Source: CAD feature listing. Evaluate the final solid. Frame: model axes, mm. A direction names the side the tool comes from. Give positions to 0.01 mm unless a question says otherwise; leave off trailing zeros. Loops run counter-clockwise (first coordinate to the right, second up) from the corner with the lowest first, then second, coordinate; pieces in that order, holes last. Notation, with made-up numbers: M 82,-6.75 L 110,-6.75 A18 cw 110,7.25 Z; hole C -1,55.5 d11. An arc over 180 degrees is marked long. Write item = value, one per line.
from build123d import *

# Parameters (mm, degrees)
ESQUISSE3_W             = 28
ESQUISSE3_H             = 20
BOSS_EXTRU_1_DEPTH      = 8
ESQUISSE4_W             = 22
ESQUISSE4_H             = 14
ENL_V_MAT_EXTRU_1_DEPTH = 6
ESQUISSE5_W             = 22
ESQUISSE5_H             = 3
ENL_V_MAT_EXTRU_2_DEPTH = 4
ESQUISSE7_R             = 1
BOSS_EXTRU_2_DEPTH      = 5
ESQUISSE9_R             = 1
ENL_V_MAT_EXTRU_3_DEPTH = 2
ESQUISSE11_R            = 1
ENL_V_MAT_EXTRU_4_DEPTH = 2


with BuildPart() as part:
    # Esquisse3 → Boss.-Extru.1 (new body)
    with BuildSketch(Plane(origin=(0, 0, 0), x_dir=(1, 0, 0), z_dir=(0, 1, 0))):
        with Locations((-14, -10)):
            Rectangle(ESQUISSE3_W, ESQUISSE3_H)
    extrude(amount=BOSS_EXTRU_1_DEPTH)

    # Esquisse4 → Enlèv. mat.-Extru.1 (cut)
    with BuildSketch(Plane(origin=(0, 8, 0), x_dir=(1, 0, 0), z_dir=(0, 1, 0))):
        with Locations((-14, -10)):
            Rectangle(ESQUISSE4_W, ESQUISSE4_H)
    extrude(amount=-ENL_V_MAT_EXTRU_1_DEPTH, mode=Mode.SUBTRACT)

    # Esquisse5 → Enlèv. mat.-Extru.2 (cut)
    with BuildSketch(Plane(origin=(0, 8, 0), x_dir=(1, 0, 0), z_dir=(0, 1, 0))):
        with Locations((-14, -18.5)):
            Rectangle(ESQUISSE5_W, ESQUISSE5_H)
    extrude(amount=-ENL_V_MAT_EXTRU_2_DEPTH, mode=Mode.SUBTRACT)

    # Esquisse7 → Boss.-Extru.2 (add)
    with BuildSketch(Plane(origin=(0, 2, 0), x_dir=(1, 0, 0), z_dir=(0, 1, 0))):
        with Locations(Location((-14, -6, 0), (0, 0, 270))):
            Circle(ESQUISSE7_R)
    extrude(amount=BOSS_EXTRU_2_DEPTH)

    # Esquisse9 → Enlèv. mat.-Extru.3 (cut)
    with BuildSketch(Plane(origin=(0, 8, 0), x_dir=(1, 0, 0), z_dir=(0, 1, 0))):
        with Locations(Location((-26.25, -1.75, 0), (0, 0, 270))):
            Circle(ESQUISSE9_R)
    enl_v_mat_extru_3 = extrude(amount=-ENL_V_MAT_EXTRU_3_DEPTH, mode=Mode.SUBTRACT)

    # Symétrie1: Enlèv. mat.-Extru.3 across plane
    add(enl_v_mat_extru_3.mirror(Plane.ZY.offset(14)), mode=Mode.SUBTRACT)

    # Esquisse11 → Enlèv. mat.-Extru.4 (cut)
    with BuildSketch(Plane(origin=(0, 8, 0), x_dir=(1, 0, 0), z_dir=(0, 1, 0))):
        with Locations(Location((-26.5, -17.5, 0), (0, 0, 270))):
            Circle(ESQUISSE11_R)
    enl_v_mat_extru_4 = extrude(amount=-ENL_V_MAT_EXTRU_4_DEPTH, mode=Mode.SUBTRACT)

    # Symétrie2: Enlèv. mat.-Extru.4 across plane
    add(enl_v_mat_extru_4.mirror(Plane.ZY.offset(14)), mode=Mode.SUBTRACT)


solid = part.part
1. First-contact query: pin 1 Ø1.6 at (x, z) = (-26, 17.5) entering from +Y; pin 2 Ø3.5 at (x, z) = (-10.5, 18) entering from +Y; pin 3 Ø1.6 at (x, z) = (-26.25, 1.75) entering from +Y; pin 4 Ø7 at (x, z) = (-11.5, 13) entering from +Y. Flat tips, straight axial feed; report the tip coordinate or a pass-through.
Derived:
pin_1 = 8
pin_2 = 4
pin_3 = 6
pin_4 = 2
2. Cut plane C-C, the plane z = 1.75. Return the cut outline in (x, y), then the cut area to 3 significant figures.
Derived:
outline = M -28,0 L 0,0 L 0,8 L -0.75,8 L -0.75,6 L -2.75,6 L -2.75,8 L -25.25,8 L -25.25,6 L -27.25,6 L -27.25,8 L -28,8 Z
area = 216 mm²
3. Material intervals for probe 1 along X at (y, z) = (7, 17.5); probe 2 along X at (y, z) = (5.25, 18.5); probe 3 along X at (y, z) = (6.9, 1.75), sorted ascending. Write a range as from..to.
Derived:
probe_1 = -28..-27.5, -25.5..-25, -3..-2.5, -0.5..0
probe_2 = -28..-25, -3..0
probe_3 = -28..-27.25, -25.25..-2.75, -0.75..0
4. Pull-direction query (X, two-part tool) for faces 4 (the flat face through (-13, 8, 2.5)), 5 (the flat face through (-14, 3, 17)), 6 (the flat face through (0, 4, 10)); classes: +X half, -X half, draft (parallel to the pull), parting line (faces both ways), or undercut.
Derived:
face_4 = draft
face_5 = undercut
face_6 = +X half
5. Cut plane B-B, the plane x = -20.5. Return the cut outline in (y, z), then the cut area to 3 significant figures.
Derived:
outline = M 0,0 L 8,0 L 8,3 L 2,3 L 2,17 L 4,17 L 4,20 L 0,20 Z
area = 64.0 mm²
6. Cut plane D-D, the plane x = -14. Return the cut outline in (y, z), then the cut area to 3 significant figures.
Derived:
outline = M 0,0 L 8,0 L 8,3 L 2,3 L 2,5 L 7,5 L 7,7 L 2,7 L 2,17 L 4,17 L 4,20 L 0,20 Z
area = 74.0 mm²
7. Reachability of faces 1 (the flat face through (-25, 5, 12)), 2 (the flat face through (-14, 3, 20)), 3 (the flat face through (-14, 7, 6)) from +Z, -Z, +X, -X, +Y, -Y: full face, straight path, thin tool, end or side. Return the list, or none.
Derived:
face_1 = +Y
face_2 = +Z, +X, -X, +Y, -Y
face_3 = +Z, +Y
8. Cut plane A-A, the plane y = 2.5. Return the cut outline in (x, z).
Derived:
outline = M -28,0 L 0,0 L 0,20 L -28,20 Z; C -14,6 d2; hole M -25,3 L -3,3 L -3,17 L -25,17 Z
